```python
from build123d import *

# Parameters (mm, degrees)
BOSS_EXTRUDE1_DEPTH             = 2
BOSS_EXTRUDE2_DEPTH             = 8
BOSS_EXTRUDE2_DIRECTION_2_REACH = 41.402
BOSS_EXTRUDE3_START             = 2
BOSS_EXTRUDE3_DEPTH             = 2
FILLET1_R                       = 3


with BuildPart() as part:
    # Sketch1 → Boss-Extrude1 (new body)
    with BuildSketch(Plane(origin=(0, 0, 0), x_dir=(1, 0, 0), z_dir=(0, 1, 0))):
        with BuildLine():
            Line((-2, 2.872281323), (-2, 5.656854249))
            ThreePointArc((-2, 5.656854249), (-3.622947325, 4.782703491), (-4.903918858, 3.457105702))
            ThreePointArc((-4.903918858, 3.457105702), (-5.994787991, 0.250033892), (-5.174767653, -3.036738339))
            Line((-5.174767653, -3.036738339), (-24.325878731, -19.106428582))
            ThreePointArc((-24.325878731, -19.106428582), (0, -30.932248369), (24.325878731, -19.106428582))
            Line((24.325878731, -19.106428582), (5.174767653, -3.036738339))
            ThreePointArc((5.174767653, -3.036738339), (5.869268357, 1.245668074), (3.495228191, 4.876820675))
            ThreePointArc((3.495228191, 4.876820675), (2.775156989, 5.319633793), (2, 5.656854249))
            Line((2, 5.656854249), (2, 2.872281323))
            ThreePointArc((2, 2.872281323), (0, -3.5), (-2, 2.872281323))
        make_face()
        with BuildLine():
            Line((21.508214625, -19.352942248), (3.889192433, -4.568827226))
            ThreePointArc((3.889192433, -4.568827226), (1.593935567, -5.784407438), (-1, -5.916079783))
            ThreePointArc((-1, -5.916079783), (-2.53570957, -5.437846722), (-3.889192433, -4.568827226))
            Line((-3.889192433, -4.568827226), (-21.508214625, -19.352942248))
            ThreePointArc((-21.508214625, -19.352942248), (0, -28.933366033), (21.508214625, -19.352942248))
        make_face(mode=Mode.SUBTRACT)
    extrude(amount=BOSS_EXTRUDE1_DEPTH)

    # Sketch2 → Boss-Extrude2 (add)
    with BuildSketch(Plane(origin=(0, 0, 0), x_dir=(1, 0, 0), z_dir=(0, 1, 0))):
        with BuildLine():
            Line((-8, 0), (-5.9, 0))
            ThreePointArc((-5.9, 0), (-5.482722017, -2.179394246), (-4.289912109, -4.050512819))
            Line((-4.289912109, -4.050512819), (-5.653884688, -5.659822253))
            ThreePointArc((-5.653884688, -5.659822253), (-7.390232659, -3.063406804), (-8, 0))
        make_face()
        with BuildLine():
            Line((8, 0), (5.9, 0))
            ThreePointArc((5.9, 0), (5.482722017, -2.179394246), (4.289912109, -4.050512819))
            Line((4.289912109, -4.050512819), (5.653884688, -5.659822253))
            ThreePointArc((5.653884688, -5.659822253), (7.390232659, -3.063406804), (8, 0))
        make_face()
        with BuildLine():
            Line((3.741396832, -4.562011589), (5.251640152, -6.034921351))
            ThreePointArc((5.251640152, -6.034921351), (0, -8), (-5.251640152, -6.034921351))
            Line((-5.251640152, -6.034921351), (-3.741396832, -4.562011589))
            ThreePointArc((-3.741396832, -4.562011589), (0, -5.9), (3.741396832, -4.562011589))
        make_face()
    extrude(amount=-BOSS_EXTRUDE2_DEPTH)

    # Boss-Extrude2 direction 2: up to this face of the body (flat: up to its plane)
    boss_extrude2_direction_2_end = Plane(part.part.faces().sort_by_distance((14.359026746, 2, 11.537912405))[0])
    # Sketch2 → Boss-Extrude2 direction 2 (add, up to the picked face)
    with BuildSketch(Plane(origin=(0, 0, 0), x_dir=(1, 0, 0), z_dir=(0, 1, 0)), mode=Mode.PRIVATE) as boss_extrude2_direction_2_sk1:
        with BuildLine():
            Line((-8, 0), (-5.9, 0))
            ThreePointArc((-5.9, 0), (-5.482722017, -2.179394246), (-4.289912109, -4.050512819))
            Line((-4.289912109, -4.050512819), (-5.653884688, -5.659822253))
            ThreePointArc((-5.653884688, -5.659822253), (-7.390232659, -3.063406804), (-8, 0))
        make_face()
    boss_extrude2_direction_2_tool1 = split(extrude(boss_extrude2_direction_2_sk1.sketch, amount=BOSS_EXTRUDE2_DIRECTION_2_REACH, mode=Mode.PRIVATE), bisect_by=boss_extrude2_direction_2_end, keep=Keep.BOTH, mode=Mode.PRIVATE)
    # Sketch2 → Boss-Extrude2 direction 2 (add, up to the picked face)
    with BuildSketch(Plane(origin=(0, 0, 0), x_dir=(1, 0, 0), z_dir=(0, 1, 0)), mode=Mode.PRIVATE) as boss_extrude2_direction_2_sk2:
        with BuildLine():
            Line((8, 0), (5.9, 0))
            ThreePointArc((5.9, 0), (5.482722017, -2.179394246), (4.289912109, -4.050512819))
            Line((4.289912109, -4.050512819), (5.653884688, -5.659822253))
            ThreePointArc((5.653884688, -5.659822253), (7.390232659, -3.063406804), (8, 0))
        make_face()
    boss_extrude2_direction_2_tool2 = split(extrude(boss_extrude2_direction_2_sk2.sketch, amount=BOSS_EXTRUDE2_DIRECTION_2_REACH, mode=Mode.PRIVATE), bisect_by=boss_extrude2_direction_2_end, keep=Keep.BOTH, mode=Mode.PRIVATE)
    # Sketch2 → Boss-Extrude2 direction 2 (add, up to the picked face)
    with BuildSketch(Plane(origin=(0, 0, 0), x_dir=(1, 0, 0), z_dir=(0, 1, 0)), mode=Mode.PRIVATE) as boss_extrude2_direction_2_sk3:
        with BuildLine():
            Line((3.741396832, -4.562011589), (5.251640152, -6.034921351))
            ThreePointArc((5.251640152, -6.034921351), (0, -8), (-5.251640152, -6.034921351))
            Line((-5.251640152, -6.034921351), (-3.741396832, -4.562011589))
            ThreePointArc((-3.741396832, -4.562011589), (0, -5.9), (3.741396832, -4.562011589))
        make_face()
    boss_extrude2_direction_2_tool3 = split(extrude(boss_extrude2_direction_2_sk3.sketch, amount=BOSS_EXTRUDE2_DIRECTION_2_REACH, mode=Mode.PRIVATE), bisect_by=boss_extrude2_direction_2_end, keep=Keep.BOTH, mode=Mode.PRIVATE)
    add(boss_extrude2_direction_2_tool1.solids().sort_by(Axis((-6.329529, 0, 2.580804), (0, 1, 0)))[0])
    add(boss_extrude2_direction_2_tool2.solids().sort_by(Axis((6.329529, 0, 2.580804), (0, 1, 0)))[0])
    add(boss_extrude2_direction_2_tool3.solids().sort_by(Axis((0, 0, 6.444232), (0, 1, 0)))[0])

    # Sketch3 → Boss-Extrude3 (add)
    with BuildSketch(Plane(origin=(0, 0, 0), x_dir=(1, 0, 0), z_dir=(0, 1, 0)).offset(BOSS_EXTRUDE3_START)):
        with BuildLine():
            Line((-8, 0), (-5.903175189, 0))
            ThreePointArc((-5.903175189, 0), (0, -5.903175189), (5.903175189, 0))
            Line((5.903175189, 0), (8, 0))
            ThreePointArc((8, 0), (0, -8), (-8, 0))
        make_face()
    extrude(amount=-BOSS_EXTRUDE3_DEPTH)

    # Fillet1
    fillet1_edges = [part.edges().sort_by_distance(p)[0] for p in [
        (24.325878731, 1, 19.106428582),
        (-24.325878731, 1, 19.106428582),
        (-21.508214625, 1, 19.352942248),
        (21.508214625, 1, 19.352942248),
        (-6.723076879, 1, 4.33592404),
        (6.723076879, 1, 4.33592404),
    ]]
    fillet(fillet1_edges, radius=FILLET1_R)


solid = part.part
```
Here's how the part is built. I have some questions about the finished solid (model axes, mm). A direction names the side the tool comes from. Give positions to 0.01 mm unless a question says otherwise; leave off trailing zeros. Order: outer loops, then holes, each group sorted by start corner. A loop starts at its lowest first (then second) coordinate and runs counter-clockwise, first axis right, second up. Notation, with made-up numbers: (19, 88) - (47, 88) arc R20 ccw to (47, 122) - close; hole circle Ø3 at (-32, -39.75). An arc over 180 degrees is marked (long way). Answer as a JSON object with one key per item and string values. Group by question number.
Item 1: If we section it at D-D on x = 17.5: Please give me the cut outline in (y, z), and give its area (3 significant figures).
Item 2: If we section it at A-A on x = 0: Please give me the cut outline in (y, z), and give its area (3 significant figures).
Item 3: If we section it at C-C on z = 13: Please give me the cut outline in (x, y), and give its area (3 significant figures).
Item 4: If we section it at B-B on y = -1.25: Please give me the cut outline in (x, z), and give its area (3 significant figures).
Item 5: Please list where these lines run through material, in increasing order: probe 1 along Y at (x, z) = (5.5, 1.5); probe 2 along X at (y, z) = (1.5, 26.5); probe 3 along X at (y, z) = (-5.75, 1.5).
Item 6: If we mould it in two halves opening along Z, with no side actions, what happens to faces 6 (the cylindrical face through (-5.494, -3.944, 2.15)), 7 (the flat face through (12.306, 0.986, 11.632)), 8 (the cylindrical face through (23.05, 1.01, 19.25)), 9 (the flat face through (2, 1, -4))? For each: pulls with the +Z half, pulls with the -Z half, needs draft (parallel to the pull), parting line crosses it, or undercut.
Item 7: For P1, Ø3, axis at x = -8, y = -2, coming from the +Z side; P2, Ø6, axis at y = -6.5, z = 10, coming from the -X side; P3, Ø4, axis at x = -5, z = 26, coming from the +Y side; P4, Ø12, axis at x = -12.5, z = 14, coming from the -Y side, each with a flat end and sliding along its axis, tell me the tip position at first contact or that it passes through.
Item 8: Which directions (+Z, -Z, +X, -X, +Y, -Y) give clear straight access to the entire face, cutting with the end or side of a thin tool? Please do faces 1 (the flat face through (15.33, 0.99, 11.56)), 2 (the cylindrical face through (-0.29, 0.99, 28.93)), 3 (the flat face through (4.96, -3.94, 4.84)), 4 (the flat face through (-2, 1, -4)), 5 (the cylindrical face through (-0.1, -3.9, 5.9)).
Result set:
{
 "1": {"outline": "(0, 13.38) - (2, 13.38) - (2, 15.99) - (0, 15.99) - close; (0, 23.04) - (2, 23.04) - (2, 25.51) - (0, 25.51) - close", "area": "10.2 mm²"},
 "2": {"outline": "(-8, 5.9) - (0, 5.9) - (0, 3.5) - (2, 3.5) - (2, 8) - (-8, 8) - close; (0, 28.93) - (2, 28.93) - (2, 30.93) - (0, 30.93) - close", "area": "29.8 mm²"},
 "3": {"outline": "(-17.05, 0) - (-13.94, 0) - (-13.94, 2) - (-17.05, 2) - close; (13.94, 0) - (17.05, 0) - (17.05, 2) - (13.94, 2) - close", "area": "12.4 mm²"},
 "4": {"outline": "(-8, 0) - (-5.9, 0) arc R5.9 cw to (-4.29, 4.05) - (-5.65, 5.66) arc R8 ccw to start; (-5.25, 6.03) - (-3.74, 4.56) arc R5.9 cw to (3.74, 4.56) - (5.25, 6.03) arc R8 ccw to start; (4.29, 4.05) arc R5.9 cw to (5.9, 0) - (8, 0) arc R8 ccw to (5.65, 5.66) - close", "area": "43.1 mm²"},
 "5": {"probe 1": "0 to 2", "probe 2": "-15.95 to -11.61, 11.61 to 15.95", "probe 3": "-7.86 to -5.71, 5.71 to 7.86"},
 "6": {"face 6": "pulls with the -Z half", "face 7": "undercut", "face 8": "parting line crosses it", "face 9": "needs draft"},
 "7": {"P1": "z = 4.66", "P2": "x = -3.87", "P3": "through", "P4": "y = 0"},
 "8": {"face 1": "-Z, +X, +Y, -Y", "face 2": "+Y, -Y", "face 3": "-Y", "face 4": "-Z, +Y, -Y", "face 5": "-Z, -Y"}
}
